from build123d import *

# Parameters (mm, degrees)
F0_W     = 11
F0_H     = 2
F1_DEPTH = 20
F2_W     = 11
F2_H     = 2
F3_DEPTH = 5
F4_W     = 11
F4_H     = 2
F5_DEPTH = 5


# Not quite as in the source:
# - ends of sketch curves that miss each other by under 0.0002 mm in the source are joined


with BuildPart() as f1:
    # F0 (on Top) → F1 (new body)
    with BuildSketch(Plane.XY):
        with BuildLine():
            ThreePointArc((0, 19), (13.4350288425, 13.4350288425), (19, 0))
            Line((19, 0), (19.3316700079, 0.9884245321))
            add(Edge.make_bspline(
                [(0, 20.9999997169), (5.0418251194, 21.0644266307), (10.6034953843, 19.0446950586), (20.5243171722, 10.6653997718), (19.9493483466, 4.7892186912), (19.3316700079, 0.9884245321)],
                knots=[0, 0, 0, 0, 0.3345544691, 0.6691089382, 0.9528969744, 0.9528969744, 0.9528969744, 0.9528969744], degree=3))
            Line((0, 20.9999997169), (0, 19))
        make_face()
        with Locations((-5.5, 20)):
            Rectangle(F0_W, F0_H)
    extrude(amount=F1_DEPTH)

    # F2 (on face) → F3 (cut)
    with BuildSketch(Plane(origin=(0, 0, 0), x_dir=(1, 0, 0), z_dir=(0, 0, -1))):
        with Locations((-5.5, -20)):
            Rectangle(F2_W, F2_H)
    extrude(amount=-F3_DEPTH, mode=Mode.SUBTRACT)

    # F4 (on face) → F5 (cut)
    with BuildSketch(Plane.XY.offset(20)):
        with Locations((-5.5, 20)):
            Rectangle(F4_W, F4_H)
    extrude(amount=-F5_DEPTH, mode=Mode.SUBTRACT)


solid = f1.part
The listing builds one solid part. Answer for the finished solid, in the listing's coordinates (mm). A direction names the side the tool comes from. Give positions to 0.01 mm unless a question says otherwise; leave off trailing zeros. Loops run counter-clockwise (first coordinate to the right, second up) from the corner with the lowest first, then second, coordinate; pieces in that order, holes last. Notation, with made-up numbers: (14, 36.25) - (55, 36.25) arc R18 ccw to (55, 58.25) - close; hole circle Ø7 at (24.5, 66.5). An arc over 180 degrees is marked (long way). Answer as a JSON object with one key per item and string values.
1. A cutting plane is placed at A-A (x = -3). Write down the section's boundary in (y, z), then the cut area to 3 significant figures.
Determined:
{"outline": "(19, 5) - (21, 5) - (21, 15) - (19, 15) - close", "area": "20.0 mm²"}
2. Find the intervals of material crossed by L1, parallel to X at y = 5, z = 9; L2, parallel to X at y = 3.25, z = 5; L3, parallel to Y at x = 17.5, z = 1.75, in increasing order. Write a range as [from, to].
Determined:
{"L1": "[18.33, 19.83]", "L2": "[18.72, 19.66]", "L3": "[7.4, 12.46]"}
3. Flat-ended cylindrical pins translate along their axes: pin 1 Ø1.6 at (y, z) = (19.5, 2) entering from -X; pin 2 Ø3 at (x, z) = (-4, 8.5) entering from -Y; pin 3 Ø0.6 at (x, y) = (-5, 20) entering from -Z; pin 4 Ø2 at (x, y) = (12.5, 11) entering from -Z. Find the tip coordinate at first contact, or state that the pin passes through.
Determined:
{"pin 1": "x = 0", "pin 2": "y = 19", "pin 3": "z = 5", "pin 4": "through"}
4. For faces 1 (the flat face through (19.164, 0.487, 9.86)), 2 (the flat face through (-6, 19, 10)), 3 (the flat face through (0, 20, 18)), 4 (the flat face through (-6, 20, 5)), determine the directions among +Z, -Z, +X, -X, +Y, -Y from which every point of the face is accessible in a straight line to the end or side of a thin tool.
Determined:
{"face 1": "+Z, -Z, +X, -Y", "face 2": "+Z, -Z, -X, -Y", "face 3": "+Z, -X, +Y, -Y", "face 4": "-Z, -X, +Y, -Y"}
